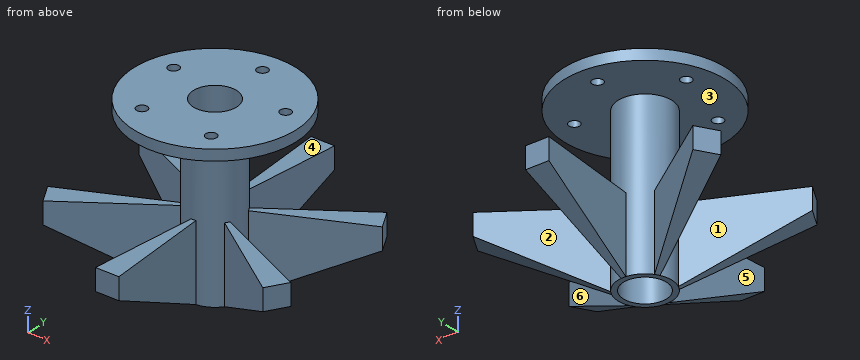
from build123d import *

# Parameters (mm, degrees)
SKETCH1_R                     = 75
SKETCH1_R_2                   = 5
BOSS_EXTRUDE1_DEPTH           = 10
SKETCH2_R                     = 25
BOSS_EXTRUDE2_DEPTH           = 150
BOSS_EXTRUDE3_DEPTH           = 70
CHAMFER2_SIZE                 = 100
CHAMFER2_SIZE2                = 50
CIRPATTERN3_COUNT             = 6
CHAMFER2_OF_CIRPATTERN3_SIZE2 = 50
CHAMFER2_OF_CIRPATTERN3_SIZE  = 100
SKETCH4_R                     = 20
CUT_EXTRUDE1_DEPTH            = 1
CUT_EXTRUDE1_DEPTH_BACK       = 161


with BuildPart() as part:
    # Sketch1 → Boss-Extrude1 (new body)
    with BuildSketch(Plane.XY):
        Circle(SKETCH1_R)
        with Locations((0, 55)):
            Circle(SKETCH1_R_2, mode=Mode.SUBTRACT)
        with Locations((52.308108396, 16.995934691)):
            Circle(SKETCH1_R_2, mode=Mode.SUBTRACT)
        with Locations((32.328188876, -44.495934691)):
            Circle(SKETCH1_R_2, mode=Mode.SUBTRACT)
        with Locations((-32.328188876, -44.495934691)):
            Circle(SKETCH1_R_2, mode=Mode.SUBTRACT)
        with Locations((-52.308108396, 16.995934691)):
            Circle(SKETCH1_R_2, mode=Mode.SUBTRACT)
    extrude(amount=BOSS_EXTRUDE1_DEPTH)

    # Sketch2 → Boss-Extrude2 (add)
    with BuildSketch(Plane(origin=(0, 0, 0), x_dir=(-1, 0, 0), z_dir=(0, 0, -1))):
        Circle(SKETCH2_R)
    extrude(amount=BOSS_EXTRUDE2_DEPTH)

    # Sketch3 → Boss-Extrude3 (add)
    with BuildSketch(Plane(origin=(0, 0, -150), x_dir=(-1, 0, 0), z_dir=(0, 0, -1))):
        with BuildLine():
            ThreePointArc((-2.178893569, 24.904867452), (0, 25), (2.178893569, 24.904867452))
            Line((2.178893569, 24.904867452), (10.927759921, 124.904867452))
            Line((10.927759921, 124.904867452), (-10.927759921, 124.904867452))
            Line((-10.927759921, 124.904867452), (-2.178893569, 24.904867452))
        make_face()
    boss_extrude3 = extrude(amount=-BOSS_EXTRUDE3_DEPTH)

    # Chamfer2
    chamfer2_edges = [part.edges().sort_by_distance(p)[0] for p in [
        (0, 124.904867452, -150),
    ]]
    chamfer2_side = [part.faces().sort_by_distance(p)[0] for p in [
        (0, 34.439140916, -150),
    ]]
    chamfer(chamfer2_edges, length=CHAMFER2_SIZE, length2=CHAMFER2_SIZE2, reference=chamfer2_side[0])

    # CirPattern3: Boss-Extrude3 ×6 about axis
    cirpattern3_axis = Axis((0, 0, 0), (0, 0, 1))
    for i in range(1, CIRPATTERN3_COUNT):
        add(boss_extrude3.rotate(cirpattern3_axis, i * 360 / CIRPATTERN3_COUNT))

    # Chamfer2 of CirPattern3
    chamfer2_of_cirpattern3_edges = [part.edges().sort_by_distance(p)[0] for p in [
        (-108.17078827, 62.452433726, -150),
        (-108.17078827, -62.452433726, -150),
        (0, -124.904867452, -150),
        (108.17078827, -62.452433726, -150),
        (108.17078827, 62.452433726, -150),
    ]]
    chamfer(chamfer2_of_cirpattern3_edges, length=CHAMFER2_OF_CIRPATTERN3_SIZE, length2=CHAMFER2_OF_CIRPATTERN3_SIZE2)

    # Sketch4 → Cut-Extrude1 (cut, two sides)
    with BuildSketch(Plane.XY.offset(10)) as cut_extrude1_sk:
        Circle(SKETCH4_R)
    extrude(amount=CUT_EXTRUDE1_DEPTH, mode=Mode.SUBTRACT)
    extrude(cut_extrude1_sk.sketch, amount=-CUT_EXTRUDE1_DEPTH_BACK, mode=Mode.SUBTRACT)


solid = part.part
Part model, mm, in its own coordinate system. Face numbers are marked on the shaded views. A direction names the side the tool comes from. Give positions to 0.01 mm unless a question says otherwise; leave off trailing zeros. Loops run counter-clockwise (first coordinate to the right, second up) from the corner with the lowest first, then second, coordinate; pieces in that order, holes last. Notation, with made-up numbers: M -7,15 L 2,15 A24 ccw 2,30 Z; hole C 80.5,64 d1. An arc over 180 degrees is marked long. Put each result on its own line as item: value. Start each with the question number.
1) Pull direction Y, two halves, no side cores. Call the marked faces 1, 2 and 3: +Y half, -Y half, draft (parallel to the pull), parting line (faces both ways), or undercut.
2) Saw through at C-C (y = -66.5). List the corners of the cut face in (x, z).
3) Flat gauge pins, fed straight in: pin 1 (18.5 mm diameter, centred on x = -68, y = 38.5, fed in from +Z); pin 2 (10 mm diameter, centred on x = 60.5, z = -122, fed in from -Y); pin 3 (2 mm diameter, centred on x = -59, z = -120.5, fed in from +Y); pin 4 (9 mm diameter, centred on x = -52.31, y = 17, fed in from -Z). Where does each tip first touch, or does it go through?
4) 3-axis set-ups, long thin cutter, end or side, ignore diameter. For the marked faces 4, 5 and 6: which of +Z, -Z, +X, -X, +Y, -Y reach the whole face in a straight line?
5) Saw through at B-B (x = 94). List the corners of the cut face in (y, z).
6) Saw through at D-D (z = -18). List the corners of the cut face in (x, y).
7) Probe probe 1 along Y at (x, z) = (0, 4); probe 2 along X at (y, z) = (-25.5, -126); probe 3 along X at (y, z) = (-10.5, -87.5). List the from-to ranges inside material, lowest first.
8) Saw through at A-A (y = 0). List the corners of the cut face in (x, z), then the cut area to 3 significant figures.
Numbers:
1. face 1: undercut
1. face 2: +Y half
1. face 3: draft
2. outline: M -105.83,-100 L -94.97,-104.7 L -94.97,-80 L -105.83,-80 Z; M -34.68,0 L 34.68,0 L 34.68,10 L -34.68,10 Z; M -5.82,-129.2 L 5.82,-129.2 L 5.82,-80 L -5.82,-80 Z; M 94.97,-104.7 L 105.83,-100 L 105.83,-80 L 94.97,-80 Z
3. pin 1: z = 10
3. pin 2: y = -45.86
3. pin 3: y = 42.01
3. pin 4: through
4. face 4: +X, -X, +Y
4. face 5: -Z
4. face 6: -Z, +X
5. outline: M -65.82,-105.29 L -43.83,-110.79 L -43.83,-80 L -65.82,-80 Z; M 43.83,-110.79 L 65.82,-105.29 L 65.82,-80 L 43.83,-80 Z
6. outline: C 0,0 d50; hole C 0,0 d40
7. probe 1: -75 to -20, 20 to 50, 60 to 75
7. probe 2: -54.68 to -36.42, -2.23 to 2.23, 36.42 to 54.68
7. probe 3: -22.69 to -17.02, 17.02 to 22.69
8. outline: M -75,0 L -25,0 L -25,-150 L -20,-150 L -20,10 L -75,10 Z; M 20,-150 L 25,-150 L 25,0 L 75,0 L 75,10 L 20,10 Z
8. area: 2,600 mm^2
